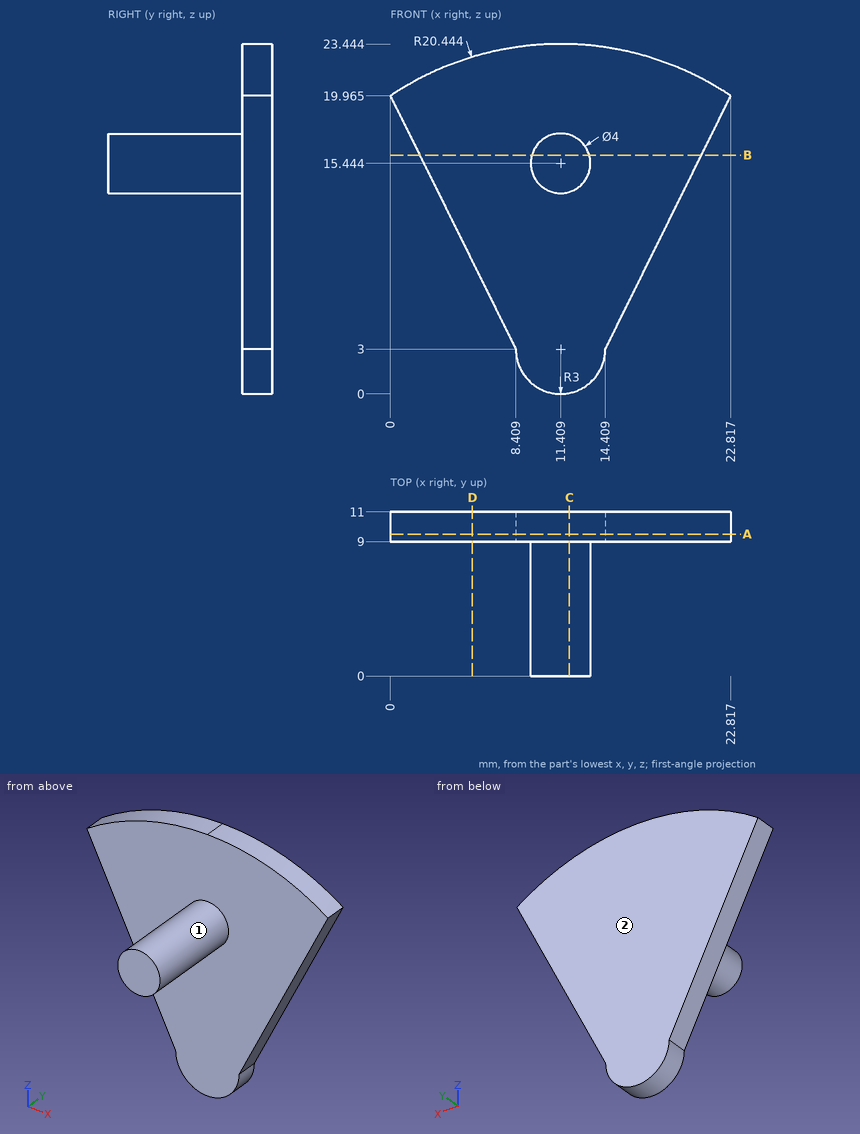
The figure shows three views and two pictorial views of one solid part (mm, origin at its lowest corner). Answer the questions. A direction names the side the tool comes from. Give positions to 0.01 mm unless a question says otherwise; leave off trailing zeros. Loops run counter-clockwise (first coordinate to the right, second up) from the corner with the lowest first, then second, coordinate; pieces in that order, holes last. Notation, with made-up numbers: (89, 85.25) -> (136, 85.25) arc R16 cw to (136, 96.25) -> close; hole circle Ø6 at (19, -16.5). An arc over 180 degrees is marked (long way). Use CSV: the item, a comma, the result in double quotes.
1. Flat-ended cylindrical pins translate along their axes: pin 1 Ø4 at (x, y) = (2.5, 9.5) entering from +Z; pin 2 Ø4 at (x, z) = (6.5, 14.5) entering from -Y; pin 3 Ø5 at (y, z) = (2.5, 16) entering from +X. Find the tip coordinate at first contact, or state that the pin passes through.
Found:
pin 1,"z = 22.24"
pin 2,"y = 9"
pin 3,"x = 13.41"
2. A tool of negligible diameter and unlimited length cuts with its end or side. For the marked faces 1 and 2, from which of +Z, -Z, +X, -X, +Y, -Y can it reach the whole face along a straight path? Write none if from no direction.
Found:
face 1,"-Y"
face 2,"+Z, -Z, +X, -X, +Y"
3. The part is cut by section B-B (z = 16). Write down the section's boundary in (x, y) (1 decimal).
Found:
outline,"(2, 9) -> (9.5, 9) -> (9.5, 0) -> (13.3, 0) -> (13.3, 9) -> (20.9, 9) -> (20.9, 11) -> (2, 11) -> close"
4. The part is cut by section A-A (y = 9.5). Write down the section's boundary in (x, z) (1 decimal).
Found:
outline,"(0, 20) -> (8.4, 3) arc R3 ccw to (14.4, 3) -> (22.8, 20) arc R20.4 ccw to start"
5. The part is cut by section D-D (x = 5.5). Write down the section's boundary in (y, z), then the cut area to 3 significant figures.
Found:
outline,"(9, 8.87) -> (11, 8.87) -> (11, 22.57) -> (9, 22.57) -> close"
area,"27.4 mm^2"
6. Straight lines are drawn through the part: line 1 (Y direction, x = 8.75, z = 14.75); line 2 (Z direction, x = 10.25, y = 2.5) (1 decimal); line 3 (X direction, y = 10.75, z = 16.25) (1 decimal). For each, find the intervals that lie inside material, in ascending order.
Found:
line 1,"9 to 11"
line 2,"13.8 to 17.1"
line 3,"1.8 to 21"
7. The part is cut by section C-C (x = 12). Write down the section's boundary in (y, z) (1 decimal).
Found:
outline,"(0, 13.5) -> (9, 13.5) -> (9, 0.1) -> (11, 0.1) -> (11, 23.4) -> (9, 23.4) -> (9, 17.4) -> (0, 17.4) -> close"
